from build123d import *

# Parameters (mm, degrees)
F1_DEPTH = 63.5
F0_W     = 25.4
F0_H     = 19.05
F0_H_2   = 4.7498
F0_H_3   = 4.7752
F2_DEPTH = 25.4


with BuildPart() as f1:
    # F0 (on Front) → F1 (new body, symmetric)
    with BuildSketch(Plane.XZ):
        Polygon((22.225, 9.525), (-41.275, 9.525), (-41.275, -9.525), (41.275, -9.525), (41.275, 9.525), align=None)
    extrude(amount=F1_DEPTH, both=True)

    # F0 (on Front) → F2 (join, symmetric)
    with BuildSketch(Plane.XZ):
        with BuildLine():
            Line((22.225, 27.0002), (22.225, 9.525))
            Line((22.225, 9.525), (41.275, 9.525))
            Line((41.275, 9.525), (41.275, 27.0002))
            ThreePointArc((41.275, 27.0002), (45.9246798487, 38.2255201513), (57.15, 42.8752))
            Line((57.15, 42.8752), (60.325, 42.8752))
            Line((60.325, 42.8752), (60.325, 61.9252))
            Line((60.325, 61.9252), (57.15, 61.9252))
            ThreePointArc((57.15, 61.9252), (32.4542956671, 51.6959043329), (22.225, 27.0002))
        make_face()
        Polygon((85.725, 66.675), (85.725, 61.9252), (85.725, 42.8752), (85.725, 38.1), (111.125, 38.1), (111.125, 66.675), align=None)
        with Locations((73.025, 52.4002)):
            Rectangle(F0_W, F0_H)
        with Locations((73.025, 64.3001)):
            Rectangle(F0_W, F0_H_2)
        with Locations((73.025, 40.4876)):
            Rectangle(F0_W, F0_H_3)
    extrude(amount=F2_DEPTH, both=True)


solid = f1.part
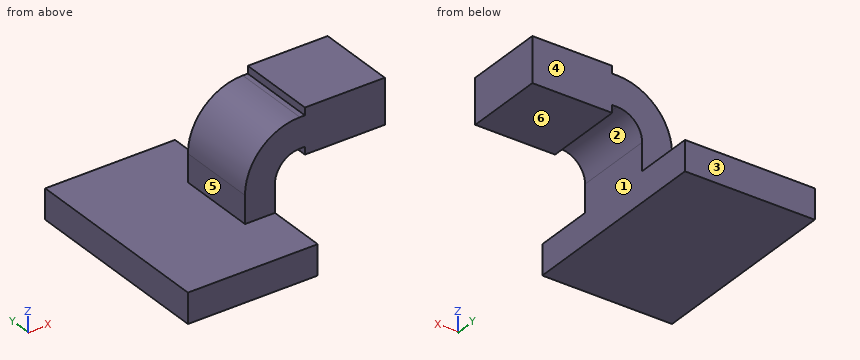
Verification items for the finished model (mm, model axes). Face numbers are marked on the shaded views. A direction names the side the tool comes from. Round coordinates to 2 decimals unless told otherwise and drop trailing zeros. Loops run counter-clockwise (first coordinate to the right, second up) from the corner with the lowest first, then second, coordinate; pieces in that order, holes last. Notation, with made-up numbers: (-40, -19) - (11, -19) arc R11 cw to (11, 2) - close; hole circle Ø3 at (42, 29.25). An arc over 180 degrees is marked (long way). Answer in a Markdown table with one row per item. Add a question column.
Q1. Section check B-B on x = 17.5. Enter the section's corners in (y, z) (3 decimals), plus the area to 3 significant figures.
Q2. Release check for a two-part mould opening along X. For the marked faces 1, 2 and 3 record: pulls with the +X half, pulls with the -X half, needs draft (parallel to the pull), parting line crosses it, or undercut.
Q3. Section check A-A on y = 0. Enter the section's corners in (x, z) (3 decimals).
Q4. Tool access check on the marked faces 4, 5 and 6. Record the directions out of +Z, -Z, +X, -X, +Y, -Y that give a thin tool (end or side, any length) a straight path to the whole face; none if there is none.
Q5. Section check C-C on z = 0. Enter the section's corners in (x, y) (3 decimals).
Q6. Gauge pin test, flat ends, axial feed: pin 1 (18.5 mm diameter, centred on y = 18.5, z = -0.5, fed in from +X) (3 decimals); pin 2 (12 mm diameter, centred on x = 61, z = 58, fed in from +Y); pin 3 (10 mm diameter, centred on x = 23.5, y = 45, fed in from +Z) (3 decimals). Record the tip position at first contact, or that the pin passes through.
Q7. Material ranges on line 1 (X direction, y = 15.5, z = 6) (3 decimals); line 2 (Z direction, x = -17, y = 47) (3 decimals); line 3 (Y direction, x = 55, z = 61), recorded low to high.
Found:
| question | item | result |
|---|---|---|
| 1 | outline | (-63.5, -9.525) - (63.5, -9.525) - (63.5, 9.525) - (-63.5, 9.525) - close |
| 1 | area | 2,420 mm² |
| 2 | face 1 | pulls with the +X half |
| 2 | face 2 | undercut |
| 2 | face 3 | needs draft |
| 3 | outline | (-41.275, -9.525) - (41.275, -9.525) - (41.275, 27) arc R15.875 cw to (57.15, 42.875) - (60.325, 42.875) - (60.325, 38.1) - (111.125, 38.1) - (111.125, 66.675) - (60.325, 66.675) - (60.325, 61.925) - (57.15, 61.925) arc R34.925 ccw to (22.225, 27) - (22.225, 9.525) - (-41.275, 9.525) - close |
| 4 | face 4 | +Z, +X, -X, +Y |
| 4 | face 5 | +Z, -X, +Y, -Y |
| 4 | face 6 | -Z, +X, +Y, -Y |
| 5 | outline | (-41.275, -63.5) - (41.275, -63.5) - (41.275, 63.5) - (-41.275, 63.5) - close |
| 6 | pin 1 | stops at x = 41.275 |
| 6 | pin 2 | stops at y = 25.4 |
| 6 | pin 3 | stops at z = 9.525 |
| 7 | line 1 | x = -41.275 to 41.275 |
| 7 | line 2 | z = -9.525 to 9.525 |
| 7 | line 3 | y = -25.4 to 25.4 |
